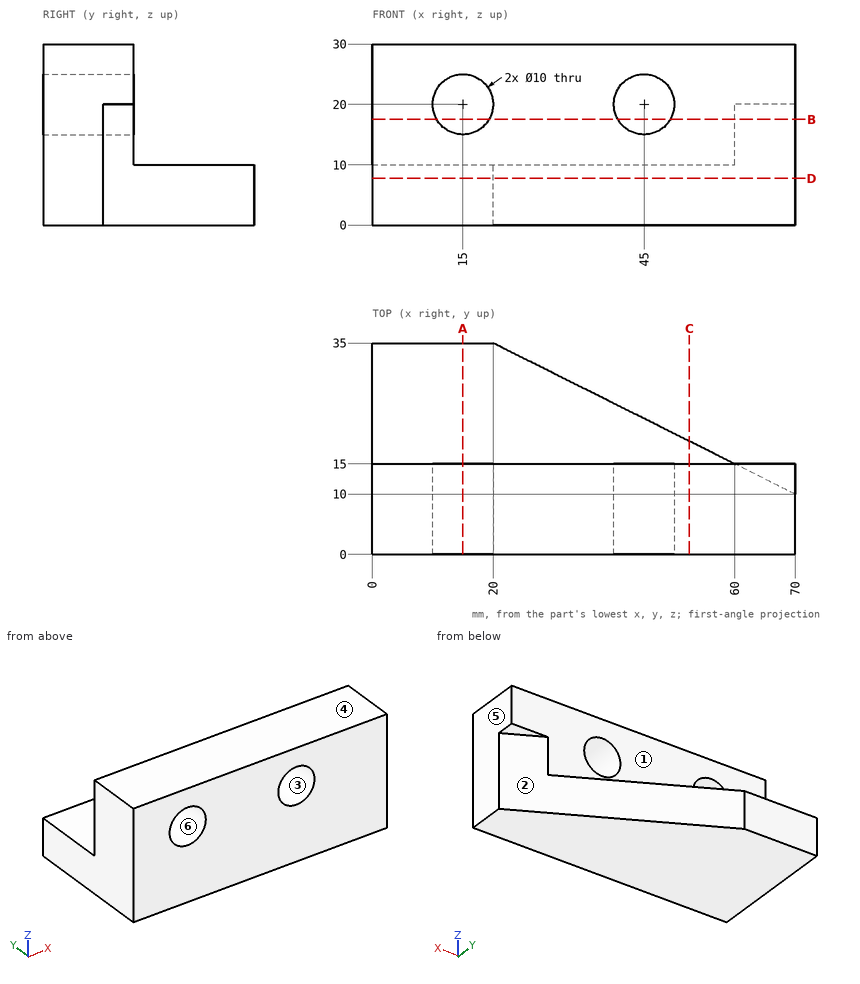
Verification items for this drawing (mm, ordinates from the low corner). A direction names the side the tool comes from. Coordinates: 2 decimals unless noted, no trailing zeros. Write each loop counter-clockwise with the first axis right and the second up, starting at its lowest first coordinate (ties: lowest second). Pieces come first, ordered by that corner, then holes. Notation, with made-up numbers: M -19.75,61.5 L 7.25,61.5 A17 ccw 7.25,76.5 Z; hole C 87,67.5 d7. An arc over 180 degrees is marked long. Answer as a JSON object with one key per item and string values.
1. Section check A-A, the plane x = 15. Enter the section's corners in (y, z).
Answers below:
{"outline": "M 0,0 L 35,0 L 35,10 L 15,10 L 15,15 L 0,15 Z; M 0,25 L 15,25 L 15,30 L 0,30 Z"}
2. Tool access check on the marked faces 1, 2 and 3. Record the directions out of +Z, -Z, +X, -X, +Y, -Y that give a thin tool (end or side, any length) a straight path to the whole face; none if there is none.
Answers below:
{"face 1": "+Z, +X, -X, +Y", "face 2": "-Z, +X, +Y", "face 3": "+Y, -Y"}
3. Go/stop test with flat-tipped pins: pin 1 Ø12 at (x, z) = (61, 14.5) entering from +Y; pin 2 Ø13 at (x, z) = (45, 20) entering from +Y; pin 3 Ø10 at (x, y) = (42, 21.5) entering from +Z. Record where each tip stops, or that it passes through.
Answers below:
{"pin 1": "stops at y = 16.48", "pin 2": "stops at y = 15", "pin 3": "stops at z = 10"}
4. Section check B-B, the plane z = 17.5. Enter the section's corners in (x, y), plus the area to 3 significant figures.
Answers below:
{"outline": "M 0,0 L 10.67,0 L 10.67,15 L 0,15 Z; M 19.33,0 L 40.67,0 L 40.67,15 L 19.33,15 Z; M 49.33,0 L 70,0 L 70,10 L 60,15 L 49.33,15 Z", "area": "765 mm²"}
5. Scan lines: L1, parallel to X at y = 5.5, z = 20; L2, parallel to Z at x = 15, y = 5.75; L3, parallel to Y at x = 65, z = 21. Record each from-to range of solid material in increasing order.
Answers below:
{"L1": "x = 0 to 10, 20 to 40, 50 to 70", "L2": "z = 0 to 15, 25 to 30", "L3": "y = 0 to 15"}
6. Draft check along X on the marked faces 4, 5 and 6. Enter one of: released by +X, released by -X, zero draft, split by the parting line, or undercut.
Answers below:
{"face 4": "zero draft", "face 5": "released by +X", "face 6": "undercut"}
7. Section check D-D, the plane z = 7.75. Enter the section's corners in (x, y), plus the area to 4 significant figures.
Answers below:
{"outline": "M 0,0 L 70,0 L 70,10 L 20,35 L 0,35 Z", "area": "1,825 mm²"}
8. Section check C-C, the plane x = 52.5. Enter the section's corners in (y, z), plus the area to 4 significant figures.
Answers below:
{"outline": "M 0,0 L 18.75,0 L 18.75,10 L 15,10 L 15,30 L 0,30 Z", "area": "487.5 mm²"}
